Check sheet for the modelled part. Datum: model origin and axes. Units: mm. Face numbers are marked on the shaded views. A direction names the side the tool comes from. Round coordinates to 2 decimals unless told otherwise and drop trailing zeros. Order: outer loops, then holes, each group sorted by start corner. A loop starts at its lowest first (then second) coordinate and runs counter-clockwise, first axis right, second up. Notation, with made-up numbers: (31, 39) -> (84, 39) arc R19 ccw to (84, 70) -> close; hole circle Ø7 at (44.5, -19). An arc over 180 degrees is marked (long way). Use CSV: the item, a comma, the result in double quotes.
Solid Edge part; units mm, degrees
sketch "Sketch1" plane through (0, 0, 0) normal (0, -1, 0) x (1, 0, 0)
  line L0 (-95, 60) -> (95, 60)
  line L1 (95, 60) -> (95, -60)
  line L2 (95, -60) -> (-95, -60)
  line L3 (-95, -60) -> (-95, 60)
  dimension "D1" = 95
  dimension "D2" = 95
extrude "Protrusion1" add sketch "Sketch1" against normal blind 15
sketch "Sketch2" plane through (0, 0, 0) normal (0, -1, 0) x (1, 0, 0)
  line L0 (-86, 20.1) -> (-14, 20.1)
  line L1 (-14, 20.1) -> (-14, -21.9)
  line L2 (-14, -21.9) -> (-86, -21.9)
  line L3 (-86, -21.9) -> (-86, 20.1)
  circle A0 centre (35, -5) radius 22
  dimension "D1" = 14
  dimension "D2" = 14
  dimension "D3" = 35
extrude "Cutout1" cut sketch "Sketch2" against normal up to vertex (15 mm away)
fillet "Redondeo_1" radius 5 4 edges at (-86, 7.5, 20.1) (-14, 7.5, 20.1) (-86, 7.5, -21.9) (-14, 7.5, -21.9)
hole "Agujero_1" at (85, 7.5, -60) direction (0, 0, 1) diameter 4.917 depth 20 tip angle 118 thread major 6 thread length 10
hole "Hole1" at (0, 7.5, -60) direction (0, 0, 1) diameter 4.917 depth 20 tip angle 118 thread major 6 thread length 10
hole "Agujero_4" at (67.5, 0, -5) direction (0, 1, 0) diameter 4.917 end up to next
pattern_circular "Pattern2" count 6 over 360 about axis through (35, 0, -5) along (0, -1, 0) of "Agujero_4"
hole "Agujero_10" at (-68.5, 0, 32.1) direction (0, 1, 0) diameter 4.917 end through all
hole "Hole7" at (-31.5, 0, 32.1) direction (0, 1, 0) diameter 4.917 end through all
hole "Hole8" at (-68.5, 0, -33.9) direction (0, 1, 0) diameter 4.917 end through all
hole "Hole9" at (-31.5, 0, -33.9) direction (0, 1, 0) diameter 4.917 end through all
chamfer "Chaflán_1" distance 50 angle 45 1 edges at (95, 7.5, 60)
sketch "Sketch3" plane through (0, 0, 0) normal (0, -1, 0) x (1, 0, 0)
  line L0 (-54, 31.1) -> (-34, 31.1)
  line L1 (-34, 31.1) -> (-34, -32.9)
  line L2 (-34, -32.9) -> (-54, -32.9)
  line L3 (-54, -32.9) -> (-54, 31.1)
  dimension "D1" = 34
  dimension "D2" = 54
extrude "Cutout2" cut sketch "Sketch3" against normal through all
fillet "Redondeo_2" radius 8 4 edges at (-34, 7.5, 31.1) (-54, 7.5, 31.1) (-54, 7.5, -32.9) (-34, 7.5, -32.9)
properties part number "1976-1200-005" material "Aluminio, 7075-T6"
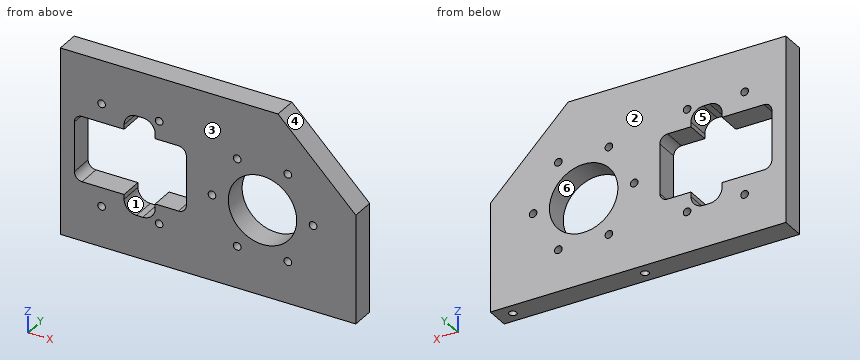
Q1. Mould release check, pull along Z, two halves, no side actions. Record for the marked faces 3, 4, 5 and 6: pulls with the +Z half, pulls with the -Z half, needs draft (parallel to the pull), parting line crosses it, or undercut.
Result sheet:
face 3,"needs draft"
face 4,"pulls with the +Z half"
face 5,"undercut"
face 6,"undercut"
Q2. Scan lines: L1, parallel to X at y = 7.5, z = -51.5; L2, parallel to X at y = 3.5, z = -16.5 (3 decimals); L3, parallel to X at y = 8.5, z = -33.9. Record each from-to range of solid material in increasing order.
Result sheet:
L1,"x = -95 to -2.46, 2.46 to 82.54, 87.46 to 95"
L2,"x = -95 to -86, -14 to 16.245, 53.755 to 95"
L3,"x = -95 to -70.96, -66.04 to -33.96, -29.04 to 16.41, 21.09 to 48.91, 53.59 to 95"
Q3. Sectioned sample at D-D, the plane x = 76.5. Enter the section's corners in (y, z).
Result sheet:
outline,"(0, -60) -> (15, -60) -> (15, 28.5) -> (0, 28.5) -> close"
Q4. Go/stop test with a flat-tipped pin: pin 1 (4 mm diameter, centred on y = 13.5, z = 23, fed in from +X). Record where the tip stops, or that it passes through.
Result sheet:
pin 1,"stops at x = 84"
Q5. Access from +Z, -Z, +X, -X, +Y, -Y to the whole of each face (thin tool, end or side, straight path). Record for the marked faces 1 and 2.
Result sheet:
face 1,"+Y, -Y"
face 2,"+Z, -Z, +X, -X, +Y"
Q6. Sectioned sample at A-A, the plane x = 35. Enter the section's corners in (y, z).
Result sheet:
outline,"(0, -60) -> (15, -60) -> (15, -27) -> (0, -27) -> close; (0, 17) -> (15, 17) -> (15, 60) -> (0, 60) -> close"
Q7. Sectioned sample at C-C, the plane z = 47.5. Enter the section's corners in (x, y), then the cut area to 3 significant figures.
Result sheet:
outline,"(-95, 0) -> (57.5, 0) -> (57.5, 15) -> (-95, 15) -> close"
area,"2,290 mm^2"
Q8. Sectioned sample at B-B, the plane x = -31.5. Enter the section's corners in (y, z).
Result sheet:
outline,"(0, -60) -> (15, -60) -> (15, -36.36) -> (0, -36.36) -> close; (0, -31.44) -> (15, -31.44) -> (15, -21.9) -> (0, -21.9) -> close; (0, 20.1) -> (15, 20.1) -> (15, 29.64) -> (0, 29.64) -> close; (0, 34.56) -> (15, 34.56) -> (15, 60) -> (0, 60) -> close"
